The listing builds one solid part. Answer for the finished solid, in the listing's coordinates (mm). Face numbers are marked on the shaded views. A direction names the side the tool comes from. Coordinates: 2 decimals unless noted, no trailing zeros. Order: outer loops, then holes, each group sorted by start corner. A loop starts at its lowest first (then second) coordinate and runs counter-clockwise, first axis right, second up. Notation, with made-up numbers: (-25.5, 62.25) - (20.5, 62.25) arc R3 ccw to (20.5, 66.25) - close; hole circle Ø7 at (-33.5, 12). An arc over 180 degrees is marked (long way). Use one line per item in the form item = value. Start each with the question number.
Item 1: Each of these flat-tipped pins is pushed along its axis until it touches: pin 1 Ø8 at (y, z) = (-9, -0.5) entering from +X; pin 2 Ø3 at (x, z) = (-15.5, 6) entering from +Y; pin 3 Ø8 at (x, z) = (9.5, 1) entering from -Y; pin 4 Ø5.5 at (x, y) = (0, 0) entering from +Z. Where does it stop, or does it pass through?
Item 2: Section D-D, the plane z = 6.5 is taken. Write down the section's boundary in (x, y) (3 decimals), and give its area (3 significant figures).
Item 3: The mould has two halves that part along Y. Classify the marked faces 1, 2 and 3: released by +Y, released by -Y, zero draft, split by the parting line, or undercut.
Item 4: A tool of negligible diameter and unlimited length cuts with its end or side. For the marked faces 4, 5, 6, 7 and 8, from which of +Z, -Z, +X, -X, +Y, -Y can it reach the whole face along a straight path? Write none if from no direction.
Item 5: Section C-C, the plane y = -5 is taken. Write down the section's boundary in (x, z).
Item 6: Section A-A, the plane x = -10 is taken. Write down the section's boundary in (y, z), and give its area (3 significant figures).
Item 7: Section B-B, the plane z = 4 is taken. Write down the section's boundary in (x, y) (3 decimals).
Item 8: Consider line 1 along Y through (x, z) = (0, 4) (3 decimals); line 2 along X through (y, z) = (-12, -4.25); line 3 along Y through (x, z) = (-10, -3.25). Determine where each line is inside the solid, lowest interval first. Write a range as [from, to].
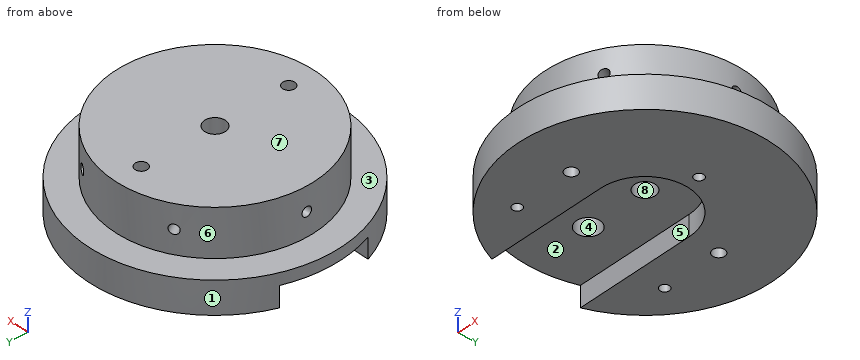
from build123d import *

# Parameters (mm, degrees)
SKETCH_1_R               = 17
EXTRUDE_1_DEPTH          = 8
SKETCH_2_R               = 21.5
EXTRUDE_2_DEPTH          = 5.5
SKETCH_3_R               = 1.75
CUT_EXTRUDE_1_DEPTH      = 34.26785235
CUT_EXTRUDE_START        = -3.5
CUT_EXTRUDE_2_DEPTH      = 3.5
SKETCH_5_R               = 1.025
CUT_EXTRUDE_3_DEPTH      = 34.26785235
SKETCH_5_3_R             = 0.8
CUT_EXTRUDE_4_DEPTH      = 8
SKETCH_6_R               = 0.8
CUT_EXTRUDE_5_DEPTH      = 3
PATTERN_CIRCULAR_1_COUNT = 6
SKETCH_7_R               = 2
CUT_EXTRUDE_6_DEPTH      = 5
SKETCH_8_R               = 0.8
CUT_EXTRUDE_7_DEPTH      = 5


with BuildPart() as part:
    # Sketch 1 → Extrude 1 (new body)
    with BuildSketch(Plane.XY):
        Circle(SKETCH_1_R)
    extrude(amount=EXTRUDE_1_DEPTH)

    # Sketch 2 → Extrude 2 (add)
    with BuildSketch(Plane(origin=(0, 0, 0), x_dir=(-1, 0, 0), z_dir=(0, 0, -1))):
        Circle(SKETCH_2_R)
    extrude(amount=EXTRUDE_2_DEPTH)

    # Sketch 3 → Cut-Extrude 1 (cut, through all)
    with BuildSketch(Plane(origin=(0, 0, -5.5), x_dir=(-1, 0, 0), z_dir=(0, 0, -1))):
        Circle(SKETCH_3_R)
    extrude(amount=-CUT_EXTRUDE_1_DEPTH, mode=Mode.SUBTRACT)

    # Sketch 4 → Cut-Extrude 2 (cut)
    with BuildSketch(Plane(origin=(0, 0, -5.5), x_dir=(-1, 0, 0), z_dir=(0, 0, -1)).offset(CUT_EXTRUDE_START)):
        with BuildLine():
            Line((0, 7.5), (20.14944168, 7.5))
            ThreePointArc((20.14944168, 7.5), (21.5, 0), (20.14944168, -7.5))
            Line((20.14944168, -7.5), (0, -7.5))
            ThreePointArc((0, -7.5), (-7.5, 0), (0, 7.5))
        make_face()
    extrude(amount=CUT_EXTRUDE_2_DEPTH, mode=Mode.SUBTRACT)

    # Sketch 5 → Cut-Extrude 3 (cut, through all)
    with BuildSketch(Plane(origin=(0, 0, -5.5), x_dir=(-1, 0, 0), z_dir=(0, 0, -1))):
        with Locations((0, -12.5)):
            Circle(SKETCH_5_R)
        with Locations(Location((0, 12.5, 0), (0, 0, 180))):
            Circle(SKETCH_5_R)
    extrude(amount=-CUT_EXTRUDE_3_DEPTH, mode=Mode.SUBTRACT)

    # Sketch 5_3 → Cut-Extrude 4 (cut)
    with BuildSketch(Plane(origin=(0, 0, -5.5), x_dir=(-1, 0, 0), z_dir=(0, 0, -1))):
        with Locations((10, -12.5)):
            Circle(SKETCH_5_3_R)
        with Locations((10, 12.5)):
            Circle(SKETCH_5_3_R)
    extrude(amount=-CUT_EXTRUDE_4_DEPTH, mode=Mode.SUBTRACT)

    # Sketch 6 → Cut-Extrude 5 (cut)
    with BuildSketch(Plane(origin=(17, 0, 0), x_dir=(0, 0, -1), z_dir=(1, 0, 0))):
        with Locations((-4, 0)):
            Circle(SKETCH_6_R)
    cut_extrude_5 = extrude(amount=-CUT_EXTRUDE_5_DEPTH, mode=Mode.SUBTRACT)

    # Pattern Circular 1: Cut-Extrude 5 ×6 about axis
    pattern_circular_1_axis = Axis((0, 0, 0), (0, 0, 1))
    for i in range(1, PATTERN_CIRCULAR_1_COUNT):
        add(cut_extrude_5.rotate(pattern_circular_1_axis, i * 360 / PATTERN_CIRCULAR_1_COUNT), mode=Mode.SUBTRACT)

    # Sketch 7 → Cut-Extrude 6 (cut)
    with BuildSketch(Plane(origin=(0, 0, -2), x_dir=(-1, 0, 0), z_dir=(0, 0, -1))):
        with Locations((10.5, 0)):
            Circle(SKETCH_7_R)
    extrude(amount=-CUT_EXTRUDE_6_DEPTH, mode=Mode.SUBTRACT)

    # Sketch 8 → Cut-Extrude 7 (cut)
    with BuildSketch(Plane(origin=(0, 0, -5.5), x_dir=(-1, 0, 0), z_dir=(0, 0, -1))):
        with Locations((-10, 0)):
            Circle(SKETCH_8_R)
    extrude(amount=-CUT_EXTRUDE_7_DEPTH, mode=Mode.SUBTRACT)


solid = part.part
Response:
q1.pin_1 = 20.91
q1.pin_2 = 9.64
q1.pin_3 = -20.75
q1.pin_4 = 8
q2.outline = circle Ø34 at (0, 0); hole circle Ø3.5 at (0, 0); hole circle Ø2.05 at (0, -12.5); hole circle Ø2.05 at (0, 12.5)
q2.area = 892 mm2
q3.face_1 = split by the parting line
q3.face_2 = undercut
q3.face_3 = zero draft
q4.face_4 = -Z
q4.face_5 = -Z, -X
q4.face_6 = +Z
q4.face_7 = +Z, +X, -X, +Y, -Y
q4.face_8 = +Z, -Z
q5.outline = (-20.91, -2) - (5.59, -2) - (5.59, -5.5) - (20.91, -5.5) - (20.91, 0) - (16.25, 0) - (16.25, 8) - (-16.25, 8) - (-16.25, 0) - (-20.91, 0) - close
q6.outline = (-19.03, -5.5) - (-13.3, -5.5) - (-13.3, 2.5) - (-11.7, 2.5) - (-11.7, -5.5) - (-7.5, -5.5) - (-7.5, -2) - (-1.94, -2) - (-1.94, 3) - (1.94, 3) - (1.94, -2) - (7.5, -2) - (7.5, -5.5) - (11.7, -5.5) - (11.7, 2.5) - (13.3, 2.5) - (13.3, -5.5) - (19.03, -5.5) - (19.03, 0) - (13.75, 0) - (13.75, 8) - (-13.75, 8) - (-13.75, 0) - (-19.03, 0) - close
q6.area = 332 mm2
q7.outline = (-16.981, -0.8) arc R17 ccw to (-9.183, -14.306) - (-7.693, -11.724) - (-6.307, -12.524) - (-7.798, -15.106) arc R17 ccw to (7.798, -15.106) - (6.307, -12.524) - (7.693, -11.724) - (9.183, -14.306) arc R17 ccw to (16.981, -0.8) - (14, -0.8) - (14, 0.8) - (16.981, 0.8) arc R17 ccw to (9.183, 14.306) - (7.693, 11.724) - (6.307, 12.524) - (7.798, 15.106) arc R17 ccw to (-7.798, 15.106) - (-6.307, 12.524) - (-7.693, 11.724) - (-9.183, 14.306) arc R17 ccw to (-16.981, 0.8) - (-14, 0.8) - (-14, -0.8) - close; hole circle Ø3.5 at (0, 0); hole circle Ø2.05 at (0, -12.5); hole circle Ø2.05 at (0, 12.5)
q8.line_1 = [-17, -13.525], [-11.475, -1.75], [1.75, 11.475], [13.525, 17]
q8.line_2 = [-17.84, -10.62], [-9.38, -0.89], [0.89, 17.84]
q8.line_3 = [-19.03, -13.3], [-11.7, -7.5], [7.5, 11.7], [13.3, 19.03]
